```python
from build123d import *

# Parameters (mm, degrees)
F0_W     = 127
F0_H     = 127
F0_W_2   = 113.03
F0_H_2   = 113.03
F1_DEPTH = 38.1
F2_W     = 113.03
F2_H     = 113.03
F3_DEPTH = 12.7
F4_R     = 5.08
F5_W     = 116.84
F5_H     = 116.84
F6_DEPTH = 12.7
F7_R     = 2.54


with BuildPart() as f1:
    # F0 (on Top) → F1 (new body)
    with BuildSketch(Plane.XY):
        Rectangle(F0_W, F0_H)
        Rectangle(F0_W_2, F0_H_2, mode=Mode.SUBTRACT)
    extrude(amount=-F1_DEPTH)

    # F2 (on Top) → F3 (join)
    with BuildSketch(Plane.XY):
        Rectangle(F2_W, F2_H)
    extrude(amount=-F3_DEPTH)

    # F4
    f4_edges = [f1.edges().sort_by_distance(p)[0] for p in [
        (-63.5, -63.5, -19.05),
        (-63.5, 63.5, -19.05),
        (63.5, 63.5, -19.05),
        (63.5, -63.5, -19.05),
    ]]
    fillet(f4_edges, radius=F4_R)

    # F5 (on face) → F6 (join)
    with BuildSketch(Plane(origin=(0, 0, -38.1), x_dir=(1, 0, 0), z_dir=(0, 0, -1))):
        with BuildLine():
            ThreePointArc((63.5, 58.42), (62.012102, 62.012102), (58.42, 63.5))
            Line((58.42, 63.5), (-58.42, 63.5))
            ThreePointArc((-58.42, 63.5), (-62.012102, 62.012102), (-63.5, 58.42))
            Line((-63.5, 58.42), (-63.5, -58.42))
            ThreePointArc((-63.5, -58.42), (-62.012102, -62.012102), (-58.42, -63.5))
            Line((-58.42, -63.5), (58.42, -63.5))
            ThreePointArc((58.42, -63.5), (62.012102, -62.012102), (63.5, -58.42))
            Line((63.5, -58.42), (63.5, 58.42))
        make_face()
        Rectangle(F5_W, F5_H, mode=Mode.SUBTRACT)
    extrude(amount=F6_DEPTH)

    # F7
    f7_edges = [f1.edges().sort_by_distance(p)[0] for p in [
        (-58.42, -58.42, -44.45),
        (58.42, -58.42, -44.45),
        (58.42, 58.42, -44.45),
        (-58.42, 58.42, -44.45),
    ]]
    fillet(f7_edges, radius=F7_R)


solid = f1.part
```
Input: part model. Units: mm. Frame: model coordinates. A direction names the side the tool comes from. Coordinates: 2 decimals unless noted, no trailing zeros. Order: outer loops, then holes, each group sorted by start corner. A loop starts at its lowest first (then second) coordinate and runs counter-clockwise, first axis right, second up. Notation, with made-up numbers: (82.25, 71) - (107.25, 71) arc R25 cw to (107.25, 86) - close; hole circle Ø9 at (74.25, 19.5). An arc over 180 degrees is marked (long way). Return JSON: item names as keys, results as strings.
Q1. First-contact query: pin 1 (5 mm diameter, centred on x = 40.5, y = 22.5, fed in from -Z). Flat tip, straight axial feed; report the tip coordinate or a pass-through.
The answers:
{"pin 1": "stops at z = -12.7"}
Q2. Draft query along Y for faces 1 (the flat face through (-1, 1, 0)), 2 (the flat face through (-1, 63.5, -25)), 3 (the flat face through (-58.42, 1, -44)). Return one class per face: +Y half, -Y half, draft (parallel to the pull), parting line (faces both ways), or undercut.
The answers:
{"face 1": "draft", "face 2": "+Y half", "face 3": "undercut"}
Q3. Ray query, probe 1 along Y at (x, z) = (36, -34) (3 decimals); probe 2 along X at (y, z) = (4.5, -39). Return the intervals inside material, ascending.
The answers:
{"probe 1": "y = -63.5 to -56.515, 56.515 to 63.5", "probe 2": "x = -63.5 to -58.42, 58.42 to 63.5"}
Q4. Access query for faces 4 (the flat face through (63.5, 1, -25)), 5 (the flat face through (-1, -56.515, -25)). Directions: +Z, -Z, +X, -X, +Y, -Y. A direction counts if a zero-diameter tool reaches every point of the face in a straight line with its end or side. Return the directions, or none.
The answers:
{"face 4": "+Z, -Z, +X, +Y, -Y", "face 5": "-Z"}
Q5. Cut plane A-A (z = -40). Return loops of the section in (x, y), then the cut area to 3 significant figures.
The answers:
{"outline": "(-63.5, -58.42) arc R5.08 ccw to (-58.42, -63.5) - (58.42, -63.5) arc R5.08 ccw to (63.5, -58.42) - (63.5, 58.42) arc R5.08 ccw to (58.42, 63.5) - (-58.42, 63.5) arc R5.08 ccw to (-63.5, 58.42) - close; hole (-58.42, -55.88) arc R2.54 ccw to (-55.88, -58.42) - (55.88, -58.42) arc R2.54 ccw to (58.42, -55.88) - (58.42, 55.88) arc R2.54 ccw to (55.88, 58.42) - (-55.88, 58.42) arc R2.54 ccw to (-58.42, 55.88) - close", "area": "2,460 mm2"}
Q6. Cut plane B-B (y = -2). Return loops of the section in (x, z) (3 decimals), then the cut area to 3 significant figures.
The answers:
{"outline": "(-63.5, -50.8) - (-58.42, -50.8) - (-58.42, -38.1) - (-56.515, -38.1) - (-56.515, -12.7) - (56.515, -12.7) - (56.515, -38.1) - (58.42, -38.1) - (58.42, -50.8) - (63.5, -50.8) - (63.5, 0) - (-63.5, 0) - close", "area": "2,100 mm2"}
